```python
from build123d import *

# Parameters (mm, degrees)
SKETCH1_W           = 80
SKETCH1_H           = 35
SKETCH1_R           = 2.5
SKETCH1_W_2         = 12
SKETCH1_H_2         = 18
SKETCH1_W_3         = 7
SKETCH1_H_3         = 12
BOSS_EXTRUDE1_DEPTH = 3
FILLET1_R           = 3


with BuildPart() as part:
    # Sketch1 → Boss-Extrude1 (new body)
    with BuildSketch(Plane(origin=(0, 0, 0), x_dir=(1, 0, 0), z_dir=(0, 1, 0))):
        with Locations((311.134650114, -80.595715333)):
            Rectangle(SKETCH1_W, SKETCH1_H)
        with Locations(Location((275.818253153, -71.268297863, 0), (0, 0, 270))):
            Circle(SKETCH1_R, mode=Mode.SUBTRACT)
        with Locations(Location((275.818253153, -91.268297863, 0), (0, 0, 270))):
            Circle(SKETCH1_R, mode=Mode.SUBTRACT)
        with Locations(Location((346.370521359, -71.268297863, 0), (0, 0, 270))):
            Circle(SKETCH1_R, mode=Mode.SUBTRACT)
        with Locations(Location((346.370521359, -91.268297863, 0), (0, 0, 270))):
            Circle(SKETCH1_R, mode=Mode.SUBTRACT)
        with Locations((315.220523964, -81.629701497)):
            Rectangle(SKETCH1_W_2, SKETCH1_H_2, mode=Mode.SUBTRACT)
        with Locations((290.062529159, -81.629701497)):
            Rectangle(SKETCH1_W_2, SKETCH1_H_2, mode=Mode.SUBTRACT)
        with Locations((335.834815931, -81.489103707)):
            Rectangle(SKETCH1_W_3, SKETCH1_H_3, mode=Mode.SUBTRACT)
    extrude(amount=BOSS_EXTRUDE1_DEPTH)

    # Fillet1
    fillet1_edges = [part.edges().sort_by_distance(p)[0] for p in [
        (271.134650114, 1.5, 63.095715333),
        (351.134650114, 1.5, 63.095715333),
        (351.134650114, 1.5, 98.095715333),
        (271.134650114, 1.5, 98.095715333),
    ]]
    fillet(fillet1_edges, radius=FILLET1_R)


solid = part.part
```
Source: CAD feature listing. Evaluate the final solid. Frame: model axes, mm. A direction names the side the tool comes from. Give positions to 0.01 mm unless a question says otherwise; leave off trailing zeros. Loops run counter-clockwise (first coordinate to the right, second up) from the corner with the lowest first, then second, coordinate; pieces in that order, holes last. Notation, with made-up numbers: (41.25, 16) - (60.25, 16) arc R29 cw to (60.25, 36) - close; hole circle Ø11 at (-22.5, 33). An arc over 180 degrees is marked (long way). Use CSV: the item, a comma, the result in double quotes.
1) Cut plane D-D (y = 1.25). Output: boundary loops of the cut face in (x, z).
Worked out:
outline,"(271.13, 66.1) arc R3 ccw to (274.13, 63.1) - (348.13, 63.1) arc R3 ccw to (351.13, 66.1) - (351.13, 95.1) arc R3 ccw to (348.13, 98.1) - (274.13, 98.1) arc R3 ccw to (271.13, 95.1) - close; hole circle Ø5 at (275.82, 71.27); hole circle Ø5 at (275.82, 91.27); hole (284.06, 72.63) - (296.06, 72.63) - (296.06, 90.63) - (284.06, 90.63) - close; hole (309.22, 72.63) - (321.22, 72.63) - (321.22, 90.63) - (309.22, 90.63) - close; hole (332.33, 75.49) - (339.33, 75.49) - (339.33, 87.49) - (332.33, 87.49) - close; hole circle Ø5 at (346.37, 71.27); hole circle Ø5 at (346.37, 91.27)"
2) Pin query (flat end, axial travel): P1, Ø3, axis at x = 302.5, z = 83.5, coming from the -Y side; P2, Ø4.5, axis at x = 346.37, z = 71.27, coming from the -Y side. Return the tip coordinate at first contact, or that it passes through.
Worked out:
P1,"stops at y = 0"
P2,"passes through"
3) Mould query, pull axis Z, two halves, no side actions, for faces 1 (the flat face through (336, 1, 75.489)), 2 (the flat face through (315, 1, 90.63)), 3 (the flat face through (271.135, 1, 81)), 4 (the cylindrical face through (350.23, 1.52, 97.24)). Classes: +Z half, -Z half, draft (parallel to the pull), parting line (faces both ways), or undercut.
Worked out:
face 1,"undercut"
face 2,"undercut"
face 3,"draft"
face 4,"+Z half"
4) Cut plane A-A (x = 311.5). Output: boundary loops of the cut face in (y, z).
Worked out:
outline,"(0, 63.1) - (3, 63.1) - (3, 72.63) - (0, 72.63) - close; (0, 90.63) - (3, 90.63) - (3, 98.1) - (0, 98.1) - close"
5) Cut plane C-C (z = 89.5). Output: boundary loops of the cut face in (x, y), and give its area (3 significant figures).
Worked out:
outline,"(271.13, 0) - (274.05, 0) - (274.05, 3) - (271.13, 3) - close; (277.59, 0) - (284.06, 0) - (284.06, 3) - (277.59, 3) - close; (296.06, 0) - (309.22, 0) - (309.22, 3) - (296.06, 3) - close; (321.22, 0) - (344.6, 0) - (344.6, 3) - (321.22, 3) - close; (348.14, 0) - (351.13, 0) - (351.13, 3) - (348.14, 3) - close"
area,"147 mm^2"
6) Line query: line 1 (X direction, y = 1.45, z = 83); line 2 (X direction, y = 2, z = 74); line 3 (Z direction, x = 288.5, y = 2.65). Output: solid intervals per line, ascending.
Worked out:
line 1,"x = 271.13 to 284.06, 296.06 to 309.22, 321.22 to 332.33, 339.33 to 351.13"
line 2,"x = 271.13 to 284.06, 296.06 to 309.22, 321.22 to 351.13"
line 3,"z = 63.1 to 72.63, 90.63 to 98.1"
7) Cut plane B-B (z = 83.5). Output: boundary loops of the cut face in (x, y).
Worked out:
outline,"(271.13, 0) - (284.06, 0) - (284.06, 3) - (271.13, 3) - close; (296.06, 0) - (309.22, 0) - (309.22, 3) - (296.06, 3) - close; (321.22, 0) - (332.33, 0) - (332.33, 3) - (321.22, 3) - close; (339.33, 0) - (351.13, 0) - (351.13, 3) - (339.33, 3) - close"
8) Set-up query: faces 5 (the cylindrical face through (350.23, 1.52, 63.95)), 6 (the flat face through (290, 1, 90.63)). Return all of +Z, -Z, +X, -X, +Y, -Y with unobstructed straight access to the full face (end or side cutting, diameter ignored); none if empty.
Worked out:
face 5,"-Z, +X, +Y, -Y"
face 6,"+Y, -Y"
